Here's how the part is built. I have some questions about the finished solid (model axes, mm). Face numbers are marked on the shaded views. A direction names the side the tool comes from. Round coordinates to 2 decimals unless told otherwise and drop trailing zeros. Write each loop counter-clockwise with the first axis right and the second up, starting at its lowest first coordinate (ties: lowest second). Pieces come first, ordered by that corner, then holes. Notation, with made-up numbers: (-18.75, 58) -> (-12.75, 58) arc R18 ccw to (-12.75, 75) -> close; hole circle Ø6 at (-31, 72.5). An arc over 180 degrees is marked (long way). Answer as CSV lines item,"result".
from build123d import *

# Parameters (mm, degrees)
PAD_DEPTH       = 6
SKETCH001_W     = 22
SKETCH001_H     = 22
POCKET_DEPTH    = 6
SKETCH002_W     = 102
SKETCH002_H     = 8
PAD001_DEPTH    = 45
SKETCH003_W     = 35
SKETCH003_H     = 17.5
POCKET001_DEPTH = 4
SKETCH004_R     = 1.5
SKETCH004_W     = 8
SKETCH004_H     = 14.5
POCKET002_DEPTH = 4
SKETCH005_W     = 20
SKETCH005_H     = 4
POCKET003_DEPTH = 15
SKETCH006_R     = 1.5
POCKET004_DEPTH = 4
PAD002_DEPTH    = 45
SKETCH008_W     = 6
SKETCH008_H     = 6
PAD003_DEPTH    = 22
SKETCH009_W     = 20
SKETCH009_H     = 5
POCKET005_DEPTH = 15
SKETCH010_R     = 1.5
POCKET006_DEPTH = 5
SKETCH011_W     = 12
SKETCH011_H     = 35
PAD004_DEPTH    = 6
SKETCH012_R     = 1.5
POCKET007_DEPTH = 12.001
POCKET008_DEPTH = 6
FILLET_R        = 2
FILLET001_R     = 2
FILLET002_R     = 2
FILLET003_R     = 2
FILLET004_R     = 2
FILLET005_R     = 2
FILLET006_R     = 2
FILLET007_R     = 1.5
FILLET008_R     = 2
FILLET009_R     = 1
FILLET010_R     = 2
FILLET011_R     = 2
FILLET012_R     = 2
FILLET013_R     = 2


with BuildPart() as part:
    # Sketch → Pad (new body)
    with BuildSketch(Plane.XY):
        Polygon((0, 0), (0, 195), (33, 195), (33, 161), (69, 161), (69, 195), (102, 195), (102, 0), align=None)
    extrude(amount=PAD_DEPTH)

    # Sketch001 (on Face10 of Pad) → Pocket (cut)
    with BuildSketch(Plane.XY.offset(6)):
        with Locations((11, 174)):
            Rectangle(SKETCH001_W, SKETCH001_H)
    extrude(amount=-POCKET_DEPTH, mode=Mode.SUBTRACT)

    # Sketch002 (on Face4 of Pocket) → Pad001 (join)
    with BuildSketch(Plane.XY.offset(6)):
        with Locations((51, 4)):
            Rectangle(SKETCH002_W, SKETCH002_H)
    extrude(amount=PAD001_DEPTH)

    # Sketch003 (on Face16 of Pad001) → Pocket001 (cut)
    with BuildSketch(Plane.XZ):
        with Locations((51, 42.25)):
            Rectangle(SKETCH003_W, SKETCH003_H)
    extrude(amount=-POCKET001_DEPTH, mode=Mode.SUBTRACT)

    # Sketch004 (on Face23 of Pocket001) → Pocket002 (cut)
    with BuildSketch(Plane.XZ.offset(-4)):
        with Locations((35.5, 35.5)):
            Circle(SKETCH004_R)
        with Locations((66.5, 35.5)):
            Circle(SKETCH004_R)
        with Locations((42.5, 43.75)):
            Rectangle(SKETCH004_W, SKETCH004_H)
    extrude(amount=-POCKET002_DEPTH, mode=Mode.SUBTRACT)

    # Sketch005 (on Face23 of Pocket002) → Pocket003 (cut)
    with BuildSketch(Plane.XY.offset(51)):
        with Locations((85.25, 2)):
            Rectangle(SKETCH005_W, SKETCH005_H)
        with Locations((16.75, 2)):
            Rectangle(SKETCH005_W, SKETCH005_H)
    extrude(amount=-POCKET003_DEPTH, mode=Mode.SUBTRACT)

    # Sketch006 (on Face36 of Pocket003) → Pocket004 (cut)
    with BuildSketch(Plane.XZ.offset(-4)):
        with Locations((16.75, 43.5)):
            Circle(SKETCH006_R)
        with Locations((85.25, 43.5)):
            Circle(SKETCH006_R)
    extrude(amount=-POCKET004_DEPTH, mode=Mode.SUBTRACT)

    # Sketch007 (on Face5 of Pocket004) → Pad002 (join)
    with BuildSketch(Plane.XY.offset(6)):
        Polygon((102, 162), (96, 162), (96, 185), (69, 185), (69, 195), (102, 195), align=None)
        Polygon((6, 162), (0, 162), (0, 195), (33, 195), (33, 185), (6, 185), align=None)
    extrude(amount=PAD002_DEPTH)

    # Sketch008 (on Face9 of Pad002) → Pad003 (join)
    with BuildSketch(Plane.XZ.offset(-185)):
        with Locations((3, 3)):
            Rectangle(SKETCH008_W, SKETCH008_H)
    extrude(amount=PAD003_DEPTH)

    # Sketch009 (on Face29 of Pad003) → Pocket005 (cut)
    with BuildSketch(Plane.XY.offset(51)):
        with Locations((16.5, 192.5)):
            Rectangle(SKETCH009_W, SKETCH009_H)
        with Locations((85.5, 192.5)):
            Rectangle(SKETCH009_W, SKETCH009_H)
    extrude(amount=-POCKET005_DEPTH, mode=Mode.SUBTRACT)

    # Sketch010 (on Face64 of Pocket005) → Pocket006 (cut)
    with BuildSketch(Plane(origin=(0, 190, 0), x_dir=(-1, 0, 0), z_dir=(0, 1, 0))):
        with Locations((-85.5, 43.5)):
            Circle(SKETCH010_R)
        with Locations((-16.5, 43.5)):
            Circle(SKETCH010_R)
    extrude(amount=-POCKET006_DEPTH, mode=Mode.SUBTRACT)

    # Sketch011 (on Face23 of Pocket006) → Pad004 (join)
    with BuildSketch(Plane.YZ.offset(6)):
        with Locations((174, 17.5)):
            Rectangle(SKETCH011_W, SKETCH011_H)
    extrude(amount=PAD004_DEPTH)

    # Sketch012 (on Face67 of Pad004) → Pocket007 (cut, through all)
    with BuildSketch(Plane.YZ.offset(12)):
        with Locations((174, 31)):
            Circle(SKETCH012_R)
    extrude(amount=-POCKET007_DEPTH, mode=Mode.SUBTRACT)

    # Sketch013 (on Face2 of Pocket007) → Pocket008 (cut)
    with BuildSketch(Plane(origin=(0, 0, 0), x_dir=(1, 0, 0), z_dir=(0, 0, -1))):
        with BuildLine():
            ThreePointArc((23.95, -69.55), (22.45, -68.05), (20.95, -69.55))
            Line((20.95, -69.55), (20.95, -139.55))
            ThreePointArc((20.95, -139.55), (22.45, -141.05), (23.95, -139.55))
            Line((23.95, -139.55), (23.95, -69.55))
        make_face()
        with BuildLine():
            ThreePointArc((81.05, -69.55), (79.55, -68.05), (78.05, -69.55))
            Line((78.05, -69.55), (78.05, -139.55))
            ThreePointArc((78.05, -139.55), (79.55, -141.05), (81.05, -139.55))
            Line((81.05, -139.55), (81.05, -69.55))
        make_face()
    extrude(amount=-POCKET008_DEPTH, mode=Mode.SUBTRACT)

    # Fillet
    fillet_edges = [part.edges().sort_by_distance(p)[0] for p in [
        (0, 81.5, 0),
    ]]
    fillet(fillet_edges, radius=FILLET_R)

    # Fillet001
    fillet001_edges = [part.edges().sort_by_distance(p)[0] for p in [
        (102, 97.5, 0),
    ]]
    fillet(fillet001_edges, radius=FILLET001_R)

    # Fillet002
    fillet002_edges = [part.edges().sort_by_distance(p)[0] for p in [
        (51, 0, 0),
    ]]
    fillet(fillet002_edges, radius=FILLET002_R)

    # Fillet003
    fillet003_edges = [part.edges().sort_by_distance(p)[0] for p in [
        (51, 0, 33.5),
        (33.5, 0, 42.25),
        (68.5, 0, 42.25),
    ]]
    fillet(fillet003_edges, radius=FILLET003_R)

    # Fillet004
    fillet004_edges = [part.edges().sort_by_distance(p)[0] for p in [
        (102, 8, 28.5),
    ]]
    fillet(fillet004_edges, radius=FILLET004_R)

    # Fillet005
    fillet005_edges = [part.edges().sort_by_distance(p)[0] for p in [
        (0, 8, 28.5),
    ]]
    fillet(fillet005_edges, radius=FILLET005_R)

    # Fillet006
    fillet006_edges = [part.edges().sort_by_distance(p)[0] for p in [
        (102, 162, 28.5),
    ]]
    fillet(fillet006_edges, radius=FILLET006_R)

    # Fillet007
    fillet007_edges = [part.edges().sort_by_distance(p)[0] for p in [
        (96, 162, 28.5),
    ]]
    fillet(fillet007_edges, radius=FILLET007_R)

    # Fillet008
    fillet008_edges = [part.edges().sort_by_distance(p)[0] for p in [
        (0, 162, 28.5),
    ]]
    fillet(fillet008_edges, radius=FILLET008_R)

    # Fillet009
    fillet009_edges = [part.edges().sort_by_distance(p)[0] for p in [
        (6, 162, 28.5),
    ]]
    fillet(fillet009_edges, radius=FILLET009_R)

    # Fillet010
    fillet010_edges = [part.edges().sort_by_distance(p)[0] for p in [
        (0, 195, 28.5),
    ]]
    fillet(fillet010_edges, radius=FILLET010_R)

    # Fillet011
    fillet011_edges = [part.edges().sort_by_distance(p)[0] for p in [
        (102, 195, 28.5),
    ]]
    fillet(fillet011_edges, radius=FILLET011_R)

    # Fillet012
    fillet012_edges = [part.edges().sort_by_distance(p)[0] for p in [
        (33, 195, 28.5),
        (69, 195, 28.5),
    ]]
    fillet(fillet012_edges, radius=FILLET012_R)

    # Fillet013
    fillet013_edges = [part.edges().sort_by_distance(p)[0] for p in [
        (51, 161, 0),
    ]]
    fillet(fillet013_edges, radius=FILLET013_R)


solid = part.part
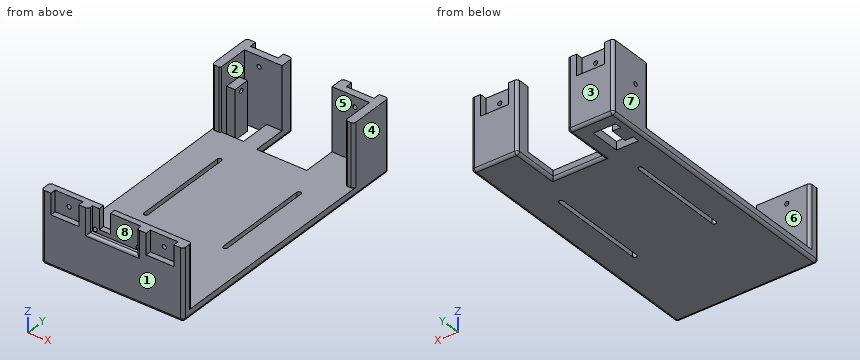
Item 1: Suppose I cut it at A-A, the plane y = 119. List the corners of the cut face in (x, z) for me, then the cut area to 3 significant figures.
Results found:
outline,"(0, 2) arc R2 ccw to (2, 0) -> (20.95, 0) -> (20.95, 6) -> (0, 6) -> close; (23.95, 0) -> (78.05, 0) -> (78.05, 6) -> (23.95, 6) -> close; (81.05, 0) -> (100, 0) arc R2 ccw to (102, 2) -> (102, 6) -> (81.05, 6) -> close"
area,"574 mm²"
Item 2: Suppose I cut it at D-D, the plane y = 19.5. List the corners of the cut face in (x, z) for me, then the cut area to 3 significant figures.
Results found:
outline,"(0, 2) arc R2 ccw to (2, 0) -> (100, 0) arc R2 ccw to (102, 2) -> (102, 6) -> (0, 6) -> close"
area,"610 mm²"
Item 3: If we mould it in two halves opening along Y, with no side actions, what happens to the marked faces 1, 2 and 3? For each: pulls with the +Y half, pulls with the -Y half, needs draft (parallel to the pull), parting line crosses it, or undercut.
Results found:
face 1,"pulls with the -Y half"
face 2,"undercut"
face 3,"pulls with the +Y half"
Item 4: Suppose I cut it at C-C, the plane x = 59.5. List the corners of the cut face in (y, z) for me, then the cut area to 3 significant figures.
Results found:
outline,"(0, 2) arc R2 ccw to (2, 0) -> (159, 0) arc R2 ccw to (161, 2) -> (161, 6) -> (8, 6) -> (8, 51) -> (4, 51) -> (4, 33.5) -> (2, 33.5) arc R2 ccw to (0, 31.5) -> close"
area,"1,250 mm²"
Item 5: I need wall thicknesses on L1, parallel to Y at x = 11, z = 21; L2, parallel to Y at x = 71.5, z = 35; L3, parallel to Z at x = 35.5, y = 7.1. Which ranges of each line are inside material? Lowest first, please.
Results found:
L1,"y = 0 to 8, 168 to 180, 185 to 195"
L2,"y = 0 to 8, 185 to 195"
L3,"z = 0 to 34, 37 to 51"
Item 6: Suppose I cut it at B-B, the plane z = 14. State how many separate pieces and enclosed holes the cut face has, then the cut area to 3 significant figures.
Results found:
separate pieces,"3"
enclosed holes,"0"
area,"1,810 mm²"
Item 7: For the marked faces 4, 5, 6, 7 and 8, which set-ups out of +Z, -Z, +X, -X, +Y, -Y let a thin tool reach every point of the face, with its end or its side?
Results found:
face 4,"+Z, -Z, +X, +Y, -Y"
face 5,"+Z"
face 6,"+Z, +X, -X"
face 7,"+Z, -Z, -X, +Y, -Y"
face 8,"+Z, -Y"
Item 8: Will these pins go through, and if not, where does the flat tip stop? pin 1 (10 mm diameter, centred on x = 90, y = 123.5, fed in from +Z); pin 2 (1 mm diameter, centred on x = 60, z = 29.5, fed in from +Y).
Results found:
pin 1,"stops at z = 6"
pin 2,"stops at y = 8"
